Autodesk Inventor part; units mm, degrees
ref_plane "YZ Plane" through (0, 0, 0) normal (1, 0, 0) x (0, 1, 0)
ref_plane "XZ Plane" through (0, 0, 0) normal (0, 1, 0) x (-1, 0, 0)
ref_plane "XY Plane" through (0, 0, 0) normal (0, 0, 1) x (1, 0, 0)
sketch "Sketch1" plane through (0, 0, 0) normal (0, 1, 0) x (-1, 0, 0)
  line L0 (0, 0) -> (-57.15, 0)
  line L1 (-57.15, 0) -> (-57.15, -41.275)
  line L2 (-57.15, -41.275) -> (0, -41.275)
  line L3 (0, -41.275) -> (0, 0)
  line L4 (-3.175, -3.175) -> (-53.975, -3.175)
  line L5 (-53.975, -3.175) -> (-53.975, -38.1)
  line L6 (-53.975, -38.1) -> (-3.175, -38.1)
  line L7 (-3.175, -38.1) -> (-3.175, -3.175)
  line L8 (0, -20.6375) -> (-57.15, -20.6375) construction
  line L9 (-28.575, 0) -> (-28.575, -41.275) construction
  point P0 (-3.175, -20.6375)
  dimension "d0" = 57.15
  dimension "d1" = 41.275
  dimension "d2" = 3.175
  dimension "d3" = 3.175
extrude "Extrusion4" add sketch "Sketch1" along normal blind 9.525
sketch "Sketch4" plane through (57.15, 0, 0) normal (1, 0, 0) x (0, 0, -1)
  line L0 (0, 0) -> (0, 9.525)
  line L1 (0, 0) -> (10.4775, 0)
  line L2 (10.4775, 0) -> (10.4775, -3.175)
  line L3 (10.4775, -3.175) -> (0, -3.175)
  line L4 (0, -3.175) -> (0, 0)
  line L5 (41.275, 0) -> (41.275, 9.525)
  line L6 (41.275, 0) -> (30.7975, 0)
  line L7 (30.7975, 0) -> (30.7975, -3.175)
  line L8 (30.7975, -3.175) -> (41.275, -3.175)
  line L9 (41.275, -3.175) -> (41.275, 0)
  line L10 (3.175, 9.525) -> (38.1, 9.525) construction
  line L11 (20.6375, 9.525) -> (20.6375, 0) construction
  line L12 (3.175, 0) -> (38.1, 0) construction
  dimension "d25" = 20.32
  dimension "d26" = 3.175
extrude "Extrusion5" add sketch "Sketch4" against normal up to surface (57.15 mm away)
sketch "Sketch5" plane through (0, 9.525, 0) normal (0, 0, 1) x (1, 0, 0)
  line L0 (57.15, -12.7) -> (0, -12.7)
  line L1 (37.465, -12.7) -> (45.085, -12.7)
  line L2 (45.085, -12.7) -> (45.085, -6.35)
  line L3 (45.085, -6.35) -> (37.465, -6.35)
  line L4 (37.465, -6.35) -> (37.465, -12.7)
  line L5 (53.975, -9.525) -> (53.975, 0)
  line L6 (0, -12.7) -> (0, 0)
  line L7 (3.175, -9.525) -> (3.175, 0)
  point P0 (0, -9.525)
  dimension "d29" = 16.51
  dimension "d31" = 41.91
  dimension "d32" = 6.35
extrude "Extrusion6" cut sketch "Sketch5" against normal up to surface (10.4775 mm away)
sketch "Sketch6" plane through (57.15, -3.175, -41.275) normal (0, -1, 0) x (1, 0, 0)
  point P0 (-57.15, 41.275)
sketch "Sketch7" plane through (57.15, -3.175, -41.275) normal (0, -1, 0) x (1, 0, 0)
  line L0 (-3.175, 10.4775) -> (0, 10.4775)
  line L1 (0, 10.4775) -> (-9.525, 10.4775)
  line L2 (-9.525, 10.4775) -> (-9.525, 7.3025)
  line L3 (-9.525, 7.3025) -> (0, 7.3025)
  line L4 (0, 7.3025) -> (0, 10.4775)
  line L5 (0, 41.275) -> (0, 0) construction
  line L6 (0, 20.6375) -> (-57.15, 20.6375) construction
  line L7 (-57.15, 0) -> (-57.15, 41.275) construction
  line L8 (0, 30.7975) -> (-9.525, 30.7975)
  line L9 (-9.525, 30.7975) -> (-9.525, 33.9725)
  line L10 (-9.525, 33.9725) -> (0, 33.9725)
  line L11 (0, 33.9725) -> (0, 30.7975)
  line L12 (0, 0) -> (-57.15, 0) construction
  line L13 (-28.575, 0) -> (-28.575, 41.275) construction
  line L14 (-19.685, 41.275) -> (-57.15, 41.275) construction
  line L15 (-57.15, 10.4775) -> (-47.625, 10.4775)
  line L16 (-47.625, 10.4775) -> (-47.625, 7.3025)
  line L17 (-47.625, 7.3025) -> (-57.15, 7.3025)
  line L18 (-57.15, 7.3025) -> (-57.15, 10.4775)
  line L19 (-57.15, 41.275) -> (-57.15, 0) construction
  line L20 (-57.15, 30.7975) -> (-47.625, 30.7975)
  line L21 (-47.625, 30.7975) -> (-47.625, 33.9725)
  line L22 (-47.625, 33.9725) -> (-57.15, 33.9725)
  line L23 (-57.15, 33.9725) -> (-57.15, 30.7975)
  dimension "d35" = 3.175
  dimension "d36" = 9.525
extrude "Extrusion7" add sketch "Sketch7" along normal blind 28.575
sketch "Sketch8" plane through (0, -3.175, -7.3025) normal (0, 0, 1) x (1, 0, 0)
  point P0 (0, 3.175)
sketch "Sketch9" plane through (0, 9.525, 0) normal (0, 0, 1) x (1, 0, 0)
  line L0 (0, -12.7) -> (0, -41.275)
  line L1 (9.525, -12.7) -> (9.525, -41.275)
  line L2 (0, -41.275) -> (9.525, -41.275)
  line L3 (9.525, -41.275) -> (9.525, -38.1)
  line L4 (9.525, -38.1) -> (0, -38.1)
  line L5 (0, -38.1) -> (0, -41.275)
  line L6 (57.15, -41.275) -> (57.15, -9.525)
  line L7 (47.625, -12.7) -> (47.625, -41.275)
  line L8 (57.15, -41.275) -> (47.625, -41.275)
  line L9 (47.625, -41.275) -> (47.625, -38.1)
  line L10 (47.625, -38.1) -> (57.15, -38.1)
  line L11 (57.15, -38.1) -> (57.15, -41.275)
  point P0 (0, -9.525)
  point P1 (0, -38.1)
  dimension "d39" = 3.175
extrude "Extrusion8" add sketch "Sketch9" against normal up to surface (41.275 mm away)
properties part number "gcs microhard"
Could you check a few things on this model? Use its own coordinates, in mm. A direction names the side the tool comes from. Round coordinates to 2 decimals unless told otherwise and drop trailing zeros. Write each loop counter-clockwise with the first axis right and the second up, starting at its lowest first coordinate (ties: lowest second). Pieces come first, ordered by that corner, then holes. Notation, with made-up numbers: M 43.25,5 L 90.25,5 A8 ccw 90.25,12 Z; hole C 7,65.25 d6. An arc over 180 degrees is marked long. Write each question's results on one line, items separated by ' | '. Start each with the question number.
1. Imagine slicing it at D-D on z = -24. List the corners of the cut face in (x, y) for me (3 decimals).
2. Imagine slicing it at A-A on y = -2.5. Count the separate pieces of the cut face and the enclosed holes in it, and give its area (3 significant figures).
3. Imagine slicing it at B-B on x = 41. List the corners of the cut face in (y, z) for me (1 decimal).
4. Imagine slicing it at C-C on z = -9. List the corners of the cut face in (x, y) for me (3 decimals).
5. On a 3-axis mill with a long thin cutter (end or side, diameter ignored), from which of +Z, -Z, +X, -X, +Y, -Y can I reach the whole of each face in a straight line? I mean faces 1 (the face through (37.465, -1, -4)), 2 (the face through (52, -28.575, -4)), 3 (the face through (19, -3.175, -5)). Say none if no direction works.
6. Thinking about a two-plate mould opening in Z: for faces 4 (the face through (29, 5, -38.1)), 5 (the face through (45.085, -1, -4)), 6 (the face through (5, -16, -7.302)), 7 (the face through (9, -11, -10.478)), which applies, +Z half, -Z half, draft (parallel to the pull), parting line (faces both ways), or undercut?
7. I need wall thicknesses on L1, parallel to X at y = 0, z = -2.5 (3 decimals); L2, parallel to Z at x = 6, y = -16; L3, parallel to X at y = 7.5, z = -17 (3 decimals). Which ranges of each line are inside material? Lowest first, please. Write a range as from..to.
8. I'm going to push flat-ended pins straight in: pin 1 Ø7.5 at (x, y) = (50.5, -16.5) entering from +Z; pin 2 Ø3.5 at (x, z) = (39.5, -33) entering from +Y; pin 3 Ø7 at (y, z) = (-1.5, -4) entering from -X; pin 4 Ø9.5 at (x, y) = (52, -8) entering from -Z. Where does each tip first touch, or does it pass through?
Result sheet:
1) outline: M 0,-31.75 L 9.525,-31.75 L 9.525,-28.575 L 0,-28.575 Z; M 0,0 L 3.175,0 L 3.175,9.525 L 0,9.525 Z; M 47.625,-31.75 L 57.15,-31.75 L 57.15,-28.575 L 47.625,-28.575 Z; M 53.975,0 L 57.15,0 L 57.15,9.525 L 53.975,9.525 Z
2) separate pieces: 3 | enclosed holes: 0 | area: 1,120 mm^2
3) outline: M -3.2,-41.3 L 9.5,-41.3 L 9.5,-38.1 L 0,-38.1 L 0,-30.8 L -3.2,-30.8 Z; M 3.2,-3.2 L 9.5,-3.2 L 9.5,0 L 3.2,0 Z
4) outline: M 0,-31.75 L 9.525,-31.75 L 9.525,-3.175 L 37.465,-3.175 L 37.465,0 L 3.175,0 L 3.175,9.525 L 0,9.525 Z; M 45.085,-3.175 L 47.625,-3.175 L 47.625,-31.75 L 57.15,-31.75 L 57.15,9.525 L 53.975,9.525 L 53.975,0 L 45.085,0 Z
5) face 1: +Z, -Y | face 2: +Z, +X, -X | face 3: +Z
6) face 4: undercut | face 5: draft | face 6: +Z half | face 7: undercut
7) L1: x = 0..37.465, 45.085..57.15 | L2: z = -33.97..-30.8, -10.48..-7.3 | L3: x = 0..3.175, 53.975..57.15
8) pin 1: stops at z = -7.3 | pin 2: stops at y = 0 | pin 3: stops at x = 0 | pin 4: stops at z = -33.97
